Solid Edge part; units mm, degrees
sketch "Sketch1" plane through (0, 0, 0) normal (0, -1, 0) x (1, 0, 0)
  line L0 (-85, 175) -> (-85, -175)
  line L1 (-85, -175) -> (85, -175)
  line L2 (85, -175) -> (85, 175)
  line L3 (85, 175) -> (-85, 175)
extrude "Protrusion1" add sketch "Sketch1" against normal blind 400
sketch "Sketch2" plane through (0, 400, 0) normal (0, 1, 0) x (1, 0, 0)
  circle A0 centre (-70, 55) radius 15
extrude "Extrusionsausprägung_9" add sketch "Sketch2" along normal blind 900
mirror "Mirror1" about plane through (0, 0, 0) normal (0, 0, 1) of "Extrusionsausprägung_9"
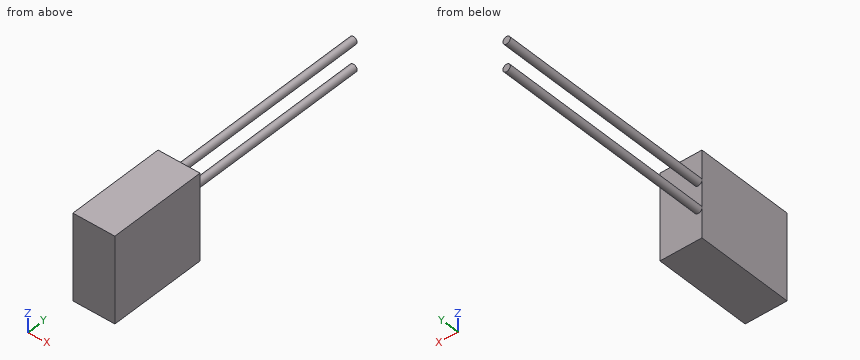
Design review of the part built by this model. Coordinates are the model's own, in mm. Round coordinates to 2 decimals unless told otherwise and drop trailing zeros. Write each loop counter-clockwise with the first axis right and the second up, starting at its lowest first coordinate (ties: lowest second). Pieces come first, ordered by that corner, then holes.
Item 1: We need section C-C on z = -125. Write out the cut boundary in (x, y).
Item 2: Clearance check with flat-ended pins moving along their axes: pin 1 Ø3 at (x, y) = (-57, 429.5) entering from -Z; pin 2 Ø6 at (x, z) = (-29.5, -109) entering from +Y. State where each tip first meets the part, or that it passes through.
Item 3: We need section B-B on y = 523. Write out the cut boundary in (x, z).
Item 4: For probe 1 along Y at (x, z) = (40.5, 19); probe 2 along Z at (x, y) = (-72.5, 536.5); probe 3 along Z at (x, y) = (-68, 1199.5), list the stretches that pass through material, from the lowest coordinate up.
Item 5: We need section D-D on x = -21.5. Write out the cut boundary in (y, z).
Item 6: We need section A-A on x = -70. Write out the cut boundary in (y, z).
Returned:
1. outline: (-85, 0) - (85, 0) - (85, 400) - (-85, 400) - close
2. pin 1: stops at z = -64.63
2. pin 2: stops at y = 400
3. outline: circle Ø30 at (-70, -55); circle Ø30 at (-70, 55)
4. probe 1: y = 0 to 400
4. probe 2: z = -69.79 to -40.21, 40.21 to 69.79
4. probe 3: z = -69.87 to -40.13, 40.13 to 69.87
5. outline: (0, -175) - (400, -175) - (400, 175) - (0, 175) - close
6. outline: (0, -175) - (400, -175) - (400, -70) - (1300, -70) - (1300, -40) - (400, -40) - (400, 40) - (1300, 40) - (1300, 70) - (400, 70) - (400, 175) - (0, 175) - close
